Autodesk Inventor part; units mm, degrees
ref_plane "YZ Plane" through (0, 0, 0) normal (1, 0, 0) x (0, 1, 0)
ref_plane "XZ Plane" through (0, 0, 0) normal (0, 1, 0) x (-1, 0, 0)
ref_plane "XY Plane" through (0, 0, 0) normal (0, 0, 1) x (1, 0, 0)
sketch "Sketch1" plane through (0, 0, 0) normal (0, 1, 0) x (-1, 0, 0)
  line L0 (20.25, -10) -> (-20.25, -10)
  line L1 (-20.25, -10) -> (-20.25, 10)
  line L2 (-20.25, 10) -> (20.25, 10)
  line L3 (20.25, 10) -> (20.25, -10)
  point P0 (0, 0)
  dimension "d0" = 40.5
  dimension "d1" = 20
  dimension "d2" = 10
  dimension "d3" = 20.25
extrude "Plate1" add sketch "Sketch1" along normal blind 1.5
sketch "Sketch2" plane through (21.75, 0, -10) normal (-1, 0, 0) x (0, -1, 0)
  line L0 (0, 20) -> (0, 0)
  line L1 (0, 0) -> (-30, 0)
  line L2 (-30, 0) -> (-30, 20)
  line L3 (-30, 20) -> (0, 20)
edge flange "Flange1" height 30 angle 90 thickness 1.5 bend radius 0.31 thickness toward (-1, 0, 0) relief tear relief width 1.5 relief depth 0.75 edges at (20.25, 1.5, 0) wall of the first edge with corners at (21.75, 0, 10) (21.75, 0, -10) (21.75, 30, -10) (21.75, 30, 10)
bend "Bend1"
corner "Corner1"
sketch "Sketch3" plane through (-21.75, 0, 10) normal (1, 0, 0) x (0, 1, 0)
  line L0 (0, -20) -> (0, 0)
  line L1 (0, 0) -> (30, 0)
  line L2 (30, 0) -> (30, -20)
  line L3 (30, -20) -> (0, -20)
edge flange "Flange2" height 30 angle 90 thickness 1.5 bend radius 0.31 thickness toward (1, 0, 0) relief tear relief width 1.5 relief depth 0.75 edges at (-20.25, 1.5, 0) wall of the first edge with corners at (-21.75, 0, -10) (-21.75, 0, 10) (-21.75, 30, 10) (-21.75, 30, -10)
bend "Bend2"
corner "Corner2"
equation "\"d4\" = Thickness"
equation "\"d5\" = BendReliefWidth"
equation "\"d6\" = BendReliefDepth"
equation "\"d7\" = MinimumRemnant"
equation "\"d8\" = TransitionRadius"
equation "\"d11\" = BendRadius"
equation "\"d12\" = CornerReliefSize"
equation "\"d13\" = GapSize"
equation "\"d14\" = JacobiRadiusSize"
equation "\"d15\" = BendReliefWidth"
equation "\"d16\" = BendReliefDepth"
equation "\"d17\" = MinimumRemnant"
equation "\"d18\" = TransitionRadius"
equation "\"d21\" = BendRadius"
equation "\"d22\" = CornerReliefSize"
equation "\"d23\" = GapSize"
equation "\"d24\" = JacobiRadiusSize"
equation "\"BendReliefWidth\" = Thickness"
equation "\"BendReliefDepth\" = 0.5 * Thickness"
equation "\"CornerReliefSize\" = 4 * Thickness"
equation "\"MinimumRemnant\" = 2 * Thickness"
equation "\"TransitionRadius\" = BendRadius"
equation "\"JacobiRadiusSize\" = BendRadius"
equation "\"GapSize\" = Thickness"
properties part number "axis_10_top_frame" material "Aluminum 6061-AHC"
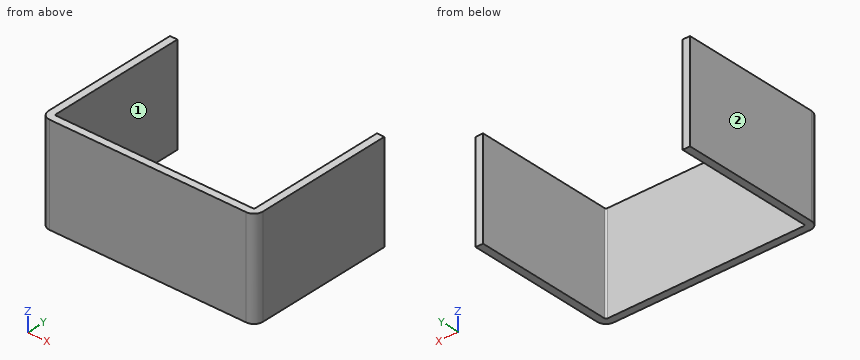
Build history of the part. All positions in model axes, mm. Face numbers are marked on the shaded views. A direction names the side the tool comes from. Round coordinates to 2 decimals unless told otherwise and drop trailing zeros. Write each loop counter-clockwise with the first axis right and the second up, starting at its lowest first coordinate (ties: lowest second). Pieces come first, ordered by that corner, then holes. Notation, with made-up numbers: M 86.25,41.5 L 112.25,41.5 A16 ccw 112.25,60.5 Z; hole C 16,65 d3. An arc over 180 degrees is marked long. Use CSV: the item, a comma, the result in double quotes.
1. Saw through at A-A (y = 17.75). Give the cut face in (x, z), plus the area to 3 significant figures.
Reply:
outline,"M -21.75,-10 L -20.25,-10 L -20.25,10 L -21.75,10 Z; M 20.25,-10 L 21.75,-10 L 21.75,10 L 20.25,10 Z"
area,"60.0 mm²"
2. Saw through at B-B (z = -6.5). Give the cut face in (x, y), plus the area to 3 significant figures.
Reply:
outline,"M -21.75,1.81 A1.81 ccw -19.94,0 L 19.94,0 A1.81 ccw 21.75,1.81 L 21.75,30 L 20.25,30 L 20.25,1.81 A0.31 cw 19.94,1.5 L -19.94,1.5 A0.31 cw -20.25,1.81 L -20.25,30 L -21.75,30 Z"
area,"149 mm²"
3. Flat gauge pin, fed straight in: pin 1 (1.5 mm diameter, centred on x = -9.5, z = 6.5, fed in from +Y). Where does the tip first touch, or does it go through?
Reply:
pin 1,"stops at y = 1.5"
4. Saw through at C-C (x = -18). Give the cut face in (y, z), plus the area to 3 significant figures.
Reply:
outline,"M 0,-10 L 1.5,-10 L 1.5,10 L 0,10 Z"
area,"30.0 mm²"
5. Wall check: probe 1 along X at (y, z) = (7.25, 7.25); probe 2 along Y at (x, z) = (-16, -4.5); probe 3 along X at (y, z) = (1.25, 5.5). Give the ranges that are in metal, low to high. Write a range as from..to.
Reply:
probe 1,"x = -21.75..-20.25, 20.25..21.75"
probe 2,"y = 0..1.5"
probe 3,"x = -21.66..21.66"
6. Tool access for the marked faces 1 and 2: list every direction of +Z, -Z, +X, -X, +Y, -Y with a clear straight run to the whole face (end or side of a thin tool).
Reply:
face 1,"+Z, -Z, +Y"
face 2,"+Z, -Z, -X, +Y, -Y"
